Source: CAD feature listing. Evaluate the final solid. Frame: model axes, mm. A direction names the side the tool comes from. Coordinates: 2 decimals unless noted, no trailing zeros. Loops run counter-clockwise (first coordinate to the right, second up) from the corner with the lowest first, then second, coordinate; pieces in that order, holes last. Notation, with made-up numbers: (39, -9) -> (73, -9) arc R10 ccw to (73, -4) -> close; hole circle Ø3 at (12, 71.5). An arc over 180 degrees is marked (long way). Answer as a JSON object with one key per item and string values. Group by question number.
from build123d import *

# Parameters (mm, degrees)
F1_DEPTH = 4
F3_DEPTH = 2.42
F4_R     = 1.55
F5_DEPTH = 25
F6_R     = 6.5
F7_DEPTH = 1
F9_DEPTH = 1.8


with BuildPart() as f1:
    # F0 (on Top) → F1 (new body)
    with BuildSketch(Plane.XY):
        Polygon((3.775, -2.179497), (3.775, 2.179497), (0, 4.358995), (-3.775, 2.179497), (-3.775, -2.179497), (0, -4.358995), align=None)
    extrude(amount=F1_DEPTH)

    # F2 (on face) → F3 (cut)
    with BuildSketch(Plane.XY.offset(4)):
        Polygon((2.8, -1.616581), (2.8, 1.616581), (0, 3.233162), (-2.8, 1.616581), (-2.8, -1.616581), (0, -3.233162), align=None)
    extrude(amount=-F3_DEPTH, mode=Mode.SUBTRACT)

    # F4 (on face) → F5 (cut)
    with BuildSketch(Plane.XY.offset(1.58)):
        Circle(F4_R)
    extrude(amount=-F5_DEPTH, mode=Mode.SUBTRACT)

    # F6 (on face) → F7 (join)
    with BuildSketch(Plane.XY.offset(4)):
        Circle(F6_R)
    extrude(amount=F7_DEPTH)

    # F8 (on face) → F9 (cut)
    with BuildSketch(Plane.XY.offset(5)):
        Polygon((2.8, -1.616581), (2.8, 1.616581), (0, 3.233162), (-2.8, 1.616581), (-2.8, -1.616581), (0, -3.233162), align=None)
    extrude(amount=-F9_DEPTH, mode=Mode.SUBTRACT)


solid = f1.part
1. Mould query, pull axis X, two halves, no side actions, for faces 1 (the face through (3, -3, 4)), 2 (the face through (-1.3, -1.4, 1.58)), 3 (the face through (0.715, -1.375, 0.801)), 4 (the face through (-1.861, 3.285, 1.972)). Classes: pulls with the +X half, pulls with the -X half, needs draft (parallel to the pull), parting line crosses it, or undercut.
2. Section query D-D on x = -3.5. Return loops of the section in (y, z).
3. Section query B-B on y = 0. Return loops of the section in (x, z) (3 decimals), then the cut area to 4 significant figures.
4. Ray query, L1, parallel to Y at x = 1, z = 0.95; L2, parallel to Z at x = 2.25, y = 3.5; L3, parallel to X at y = -0.5, z = 0.55 (3 decimals). Return the intervals inside material, ascending.
5. Reachability of faces 5 (the face through (-3.775, 0, 2)), 6 (the face through (-1.914, -3.254, 1.972)), 7 (the face through (-1.38, 2.436, 3.314)) from +Z, -Z, +X, -X, +Y, -Y: full face, straight path, thin tool, end or side. Return the list, or none.
6. Pin query (flat end, axial travel): pin 1 Ø2.5 at (x, y) = (0, 0) entering from -Z; pin 2 Ø3 at (y, z) = (-1, 2) entering from -X (3 decimals); pin 3 Ø2 at (x, z) = (-2.5, 2.5) entering from -Y; pin 4 Ø1.6 at (y, z) = (-0.5, 2.5) entering from +X (3 decimals). Return the tip coordinate at first contact, or that it passes through.
7. Section query C-C on x = -0.25. Return loops of the section in (y, z).
Solved:
{
 "1": {"face 1": "needs draft", "face 2": "undercut", "face 3": "undercut", "face 4": "pulls with the -X half"},
 "2": {"outline": "(-5.48, 4) -> (-2.34, 4) -> (-2.34, 0) -> (2.34, 0) -> (2.34, 4) -> (5.48, 4) -> (5.48, 5) -> (-5.48, 5) -> close"},
 "3": {"outline": "(-6.5, 4) -> (-3.775, 4) -> (-3.775, 0) -> (-1.55, 0) -> (-1.55, 1.58) -> (-2.8, 1.58) -> (-2.8, 5) -> (-6.5, 5) -> close; (1.55, 0) -> (3.775, 0) -> (3.775, 4) -> (6.5, 4) -> (6.5, 5) -> (2.8, 5) -> (2.8, 1.58) -> (1.55, 1.58) -> close", "area": "19.15 mm^2"},
 "4": {"L1": "-3.78 to -1.18, 1.18 to 3.78", "L2": "4 to 5", "L3": "-3.775 to -1.467, 1.467 to 3.775"},
 "5": {"face 5": "-Z, -X, +Y, -Y", "face 6": "-Z, -X, -Y", "face 7": "+Z"},
 "6": {"pin 1": "through", "pin 2": "x = -3.775", "pin 3": "y = -3.49", "pin 4": "x = 3.775"},
 "7": {"outline": "(-6.5, 4) -> (-4.21, 4) -> (-4.21, 0) -> (-1.53, 0) -> (-1.53, 1.58) -> (-3.09, 1.58) -> (-3.09, 5) -> (-6.5, 5) -> close; (1.53, 0) -> (4.21, 0) -> (4.21, 4) -> (6.5, 4) -> (6.5, 5) -> (3.09, 5) -> (3.09, 1.58) -> (1.53, 1.58) -> close"}
}
